```python
from build123d import *

# Parameters (mm, degrees)
SKETCH_W        = 50
SKETCH_H        = 15
PAD_DEPTH       = 6
SKETCH001_R     = 7
POCKET_DEPTH    = 15.001
SKETCH002_R     = 1.3
POCKET001_DEPTH = 6.001
SKETCH018_R     = 3
POCKET013_DEPTH = 4


with BuildPart() as part:
    # Sketch → Pad (new body)
    with BuildSketch(Plane.XY):
        Rectangle(SKETCH_W, SKETCH_H)
    extrude(amount=PAD_DEPTH)

    # Sketch001 (on Face3 of Pad) → Pocket (cut, through all)
    with BuildSketch(Plane.XZ.offset(7.5)):
        with Locations((0, 9)):
            Circle(SKETCH001_R)
    extrude(amount=-POCKET_DEPTH, mode=Mode.SUBTRACT)

    # Sketch002 (on Face6 of Pad) → Pocket001 (cut, through all)
    with BuildSketch(Plane.XY.offset(6)):
        with Locations((-20, 0)):
            Circle(SKETCH002_R)
        with Locations((20, 0)):
            Circle(SKETCH002_R)
    extrude(amount=-POCKET001_DEPTH, mode=Mode.SUBTRACT)

    # Sketch018 (on Face2 of Pocket001) → Pocket013 (cut)
    with BuildSketch(Plane(origin=(0, 0, 0), x_dir=(1, 0, 0), z_dir=(0, 0, -1))):
        with Locations((-20, 0)):
            Circle(SKETCH018_R)
        with Locations((20, 0)):
            Circle(SKETCH018_R)
    extrude(amount=-POCKET013_DEPTH, mode=Mode.SUBTRACT)


with BuildPart() as part_1:
    # Body placement: moved
    add(part.part.moved(Location((80, 0, 0))))


solid = part_1.part
```
Here's how the part is built. I have some questions about the finished solid (model axes, mm). A direction names the side the tool comes from. Coordinates: 2 decimals unless noted, no trailing zeros. Write each loop counter-clockwise with the first axis right and the second up, starting at its lowest first coordinate (ties: lowest second). Pieces come first, ordered by that corner, then holes. Notation, with made-up numbers: (32.25, 8.25) -> (47.25, 8.25) arc R29 cw to (47.25, 32.25) -> close; hole circle Ø10 at (60, 80). An arc over 180 degrees is marked (long way). Use a Markdown table: item, result. Add a question column.
(1) If we section it at B-B, the plane y = 0: Write out the boundary of the cut face in (x, z).
(2) Please list where these lines run through material, in increasing order: line 1 (Y direction, x = 100, z = 5.3); line 2 (Y direction, x = 60, z = 2.7); line 3 (X direction, y = 2.75, z = 0.75).
(3) We'd pull the mould along Y, two halves only. Please class faces 1 (the flat face through (64, 0, 6)), 2 (the flat face through (79.6, -7.5, 1.6)), 3 (the flat face through (79.6, 7.5, 1.6)), 4 (the cylindrical face through (61.24, 0.39, 5.01)): +Y half, -Y half, draft (parallel to the pull), parting line (faces both ways), or undercut.
(4) For faces 5 (the flat face through (55, 0, 3)), 6 (the cylindrical face through (97, 0, 2)), which set-ups out of +Z, -Z, +X, -X, +Y, -Y let a thin tool reach every point of the face, with its end or its side?
(5) If we section it at C-C, the plane x = 60: Write out the boundary of the cut face in (y, z), and give its area (3 significant figures).
(6) If we section it at A-A, the plane z = 3.5: Write out the boundary of the cut face in (x, y).
(7) If we section it at D-D, the plane z = 1: Write out the boundary of the cut face in (x, y).
(8) I'm going to push flat-ended pins straight in: P1, Ø3, axis at x = 100, y = -0.5, coming from the -Z side; P2, Ø5, axis at x = 79.5, y = 5, coming from the +Z side; P3, Ø7, axis at x = 100, y = 0, coming from the +Z side. Where does each tip first touch, or does it pass through?
Outcome:
| question | item | result |
|---|---|---|
| 1 | outline | (55, 0) -> (57, 0) -> (57, 4) -> (58.7, 4) -> (58.7, 6) -> (55, 6) -> close; (61.3, 4) -> (63, 4) -> (63, 0) -> (97, 0) -> (97, 4) -> (98.7, 4) -> (98.7, 6) -> (86.32, 6) arc R7 cw to (73.68, 6) -> (61.3, 6) -> close; (101.3, 4) -> (103, 4) -> (103, 0) -> (105, 0) -> (105, 6) -> (101.3, 6) -> close |
| 2 | line 1 | y = -7.5 to -1.3, 1.3 to 7.5 |
| 2 | line 2 | y = -7.5 to -3, 3 to 7.5 |
| 2 | line 3 | x = 55 to 58.8, 61.2 to 98.8, 101.2 to 105 |
| 3 | face 1 | draft |
| 3 | face 2 | -Y half |
| 3 | face 3 | +Y half |
| 3 | face 4 | undercut |
| 4 | face 5 | +Z, -Z, -X, +Y, -Y |
| 4 | face 6 | -Z |
| 5 | outline | (-7.5, 0) -> (-3, 0) -> (-3, 4) -> (-1.3, 4) -> (-1.3, 6) -> (-7.5, 6) -> close; (1.3, 4) -> (3, 4) -> (3, 0) -> (7.5, 0) -> (7.5, 6) -> (1.3, 6) -> close |
| 5 | area | 60.8 mm^2 |
| 6 | outline | (55, -7.5) -> (75.67, -7.5) -> (75.67, 7.5) -> (55, 7.5) -> close; (84.33, -7.5) -> (105, -7.5) -> (105, 7.5) -> (84.33, 7.5) -> close; hole circle Ø6 at (60, 0); hole circle Ø6 at (100, 0) |
| 7 | outline | (55, -7.5) -> (105, -7.5) -> (105, 7.5) -> (55, 7.5) -> close; hole circle Ø6 at (60, 0); hole circle Ø6 at (100, 0) |
| 8 | P1 | stops at z = 4 |
| 8 | P2 | stops at z = 2.68 |
| 8 | P3 | stops at z = 6 |
